```python
from build123d import *

# Parameters (mm, degrees)
BOSS_EXTRUDE2_DEPTH = 2.54
BOSS_EXTRUDE3_DEPTH = 12.7
CUT_EXTRUDE1_DEPTH  = 13.97
FILLET1_R           = 3.8099999999999996


with BuildPart() as part:
    # Sketch1 → Boss-Extrude2 (new body)
    with BuildSketch(Plane(origin=(0, 0, 0), x_dir=(1, 0, 0), z_dir=(0, 1, 0))):
        Polygon((49.12673440534523, 7.27e-15), (24.56336720267261, 42.545), (-24.56336720267263, 42.544999999999995), (-49.12673440534525, -4.56e-15), (-24.56336720267264, -42.545), (24.56336720267261, -42.545), align=None)
        Polygon((-23.09689751893098, 40.004999999999995), (-24.56336720267272, 37.465000000000906), (-21.263810414254024, 35.560000000000905), (-39.522768565701696, 3.9345567884195773), (-38.42291630289545, 3.299556788419578), (-20.163958151447684, 34.925), (-20.163958151447687, 38.735), (16.353958151447667, 38.735), (16.353958151447667, 40.004999999999995), align=None, mode=Mode.SUBTRACT)
        Polygon((20.1639581514492, -34.92499999999734), (38.42291630289649, -3.299556788416705), (39.52276856570363, -3.934556788417227), (21.263810414255218, -35.55999999999977), (24.56336720267305, -37.464999999999264), (23.096897518930962, -40.004999999999995), (-16.353958151447596, -40.0049999999992), (-16.353958151447596, -38.7350000000008), (20.1639581514492, -38.7350000000008), align=None, mode=Mode.SUBTRACT)
        Polygon((40.32791630289463, 1.40742e-12), (22.06895815144691, 31.625443211581366), (23.168810414254217, 32.26044321158198), (41.42776856570169, 0.6350000000010452), (44.727325354119536, 2.540000000000058), (46.19379503786194, 0), (26.468367202673054, -34.16544321158055), (25.368514939866817, -33.53044321158055), (43.62747309131447, -1.9049999999993157), align=None, mode=Mode.SUBTRACT)
        Polygon((20.16395815144767, 34.925), (-16.35395815144768, 34.925), (-16.35395815144768, 36.195), (20.16395815144767, 36.195), (20.163958151447673, 40.004999999999995), (23.096897518930962, 40.004999999999995), (42.82232535411953, 5.839556788418761), (41.7224730913133, 5.204556788418767), (23.4635149398656, 36.83000000000007), align=None, mode=Mode.SUBTRACT)
        Polygon((-40.32791630289535, 3.53e-15), (-22.068958151447685, -31.6254432115805), (-23.168810414253926, -32.26044321158051), (-41.427768565701626, -0.634999999999201), (-44.72732535412034, -2.5399999999991967), (-46.19379503786196, -8.7e-16), (-26.468367202672724, 34.16544321158219), (-25.368514939866504, 33.530443211582195), (-43.62747309131417, 1.9050000000008698), align=None, mode=Mode.SUBTRACT)
        Polygon((-20.163958151444543, -34.92499999999999), (16.35395815144779, -34.924999999999194), (16.353958151447785, -36.19500000000081), (-20.1639581514476, -36.19500000000081), (-20.1639581514476, -40.00499999999919), (-23.09689751893098, -40.004999999999995), (-42.82232535412034, -5.839556788417916), (-41.72247309131411, -5.204556788417918), (-23.46351493986529, -36.83000000000117), align=None, mode=Mode.SUBTRACT)
    extrude(amount=BOSS_EXTRUDE2_DEPTH)

    # Sketch2 → Boss-Extrude3 (add)
    with BuildSketch(Plane(origin=(0, 2.54, 0), x_dir=(1, 0, 0), z_dir=(0, 1, 0))):
        Polygon((-20.163958151447684, 34.925), (-40.32791630289537, -2.429e-14), (-20.163958151447673, -34.92500000000001), (20.163958151447694, -34.92500000000001), (40.32791630289537, 2.74e-15), (20.163958151447677, 34.925), align=None)
    extrude(amount=BOSS_EXTRUDE3_DEPTH)

    # Sketch3 → Cut-Extrude1 (cut)
    with BuildSketch(Plane.XZ):
        Polygon((17.23101878396438, -29.844999999999995), (34.46203756792874, 9.8e-15), (17.231018783964352, 29.845000000000006), (-17.231018783964387, 29.845000000000002), (-34.46203756792876, -6.96e-15), (-17.231018783964384, -29.84499999999999), align=None)
    extrude(amount=-CUT_EXTRUDE1_DEPTH, mode=Mode.SUBTRACT)

    # Fillet1
    fillet1_edges = [part.edges().sort_by_distance(p)[0] for p in [
        (20.163958151447677, 8.89, -34.925),
        (-20.163958151447684, 8.89, -34.925),
        (-40.32791630289537, 8.89, 2.429e-14),
        (-20.163958151447673, 8.89, 34.92500000000001),
        (20.163958151447694, 8.89, 34.92500000000001),
        (40.32791630289537, 8.89, -2.74e-15),
        (-3.55e-15, 15.239999999999998, -34.925),
        (-30.245937227171524, 15.239999999999998, -17.462499999999988),
        (-30.24593722717152, 15.239999999999998, 17.46250000000002),
        (1.066e-14, 15.239999999999998, 34.92500000000001),
        (30.24593722717153, 15.239999999999998, 17.462500000000006),
        (30.245937227171524, 15.239999999999998, -17.462500000000002),
    ]]
    fillet(fillet1_edges, radius=FILLET1_R)


solid = part.part
```
Input: part model. Units: mm. Frame: model coordinates. A direction names the side the tool comes from. Give positions to 0.01 mm unless a question says otherwise; leave off trailing zeros. Order: outer loops, then holes, each group sorted by start corner. A loop starts at its lowest first (then second) coordinate and runs counter-clockwise, first axis right, second up.
1. Section A-A on x = -14.5. Return the cut outline in (y, z) (3 decimals), and give its area (3 significant figures).
Derived:
outline: (0, -42.545) - (2.54, -42.545) - (2.54, -40.005) - (0, -40.005) - close; (0, -38.735) - (2.54, -38.735) - (2.54, -36.195) - (0, -36.195) - close; (0, -34.925) - (11.43, -34.925) arc R3.81 ccw to (15.24, -31.115) - (15.24, 31.115) arc R3.81 ccw to (11.43, 34.925) - (0, 34.925) - (0, 29.845) - (13.97, 29.845) - (13.97, -29.845) - (0, -29.845) - close; (0, 36.195) - (2.54, 36.195) - (2.54, 38.735) - (0, 38.735) - close; (0, 40.005) - (2.54, 40.005) - (2.54, 42.545) - (0, 42.545) - close
area: 250 mm2
2. Reachability of faces 1 (the cylindrical face through (0.251, 14.154, 33.779)), 2 (the flat face through (-2, 1, -38.735)), 3 (the cylindrical face through (19.845, 7.047, -34.428)), 4 (the flat face through (-25.726, 6.887, 15.131)) from +Z, -Z, +X, -X, +Y, -Y: full face, straight path, thin tool, end or side. Return the list, or none.
Derived:
face 1: +Z, +X, -X, +Y
face 2: +Y, -Y
face 3: -Z, +X, +Y
face 4: -Y
3. Pin query (flat end, axial travel): pin 1 (1 mm diameter, centred on y = 1.5, z = -39.5, fed in from -X); pin 2 (1 mm diameter, centred on y = 2, z = -35.5, fed in from +X); pin 3 (1.5 mm diameter, centred on y = 3.5, z = -12.5, fed in from +X). Return the tip coordinate at first contact, or that it passes through.
Derived:
pin 1: stops at x = -26.61
pin 2: stops at x = 28.92
pin 3: stops at x = 33.54
4. Material intervals for L1, parallel to Z at x = -5, y = 4.75 (3 decimals); L2, parallel to Y at x = 14, z = -13; L3, parallel to X at y = 2.5, z = -6.5, sorted ascending.
Derived:
L1: z = -34.925 to -29.845, 29.845 to 34.925
L2: y = 13.97 to 15.24
L3: x = -45.37 to -42.44, -40.97 to -38.04, -36.58 to -30.71, 30.71 to 36.58, 38.04 to 40.97, 42.44 to 45.37
5. Section B-B on y = 6.25. Return the cut outline in (x, z) (1 decimal), and give its area (3 significant figures).
Derived:
outline: (-39.2, -1.9) - (-21.3, -33) arc R3.8 ccw to (-18, -34.9) - (18, -34.9) arc R3.8 ccw to (21.3, -33) - (39.2, -1.9) arc R3.8 ccw to (39.2, 1.9) - (21.3, 33) arc R3.8 ccw to (18, 34.9) - (-18, 34.9) arc R3.8 ccw to (-21.3, 33) - (-39.2, 1.9) arc R3.8 ccw to start; hole (-34.5, 0) - (-17.2, -29.8) - (17.2, -29.8) - (34.5, 0) - (17.2, 29.8) - (-17.2, 29.8) - close
area: 1,140 mm2
6. Section C-C on z = 25. Give the number of separate pieces and of enclosed holes in the cut face, and give its area (3 significant figures).
Derived:
separate pieces: 5
enclosed holes: 0
area: 252 mm2
7. Mould query, pull axis Z, two halves, no side actions, for faces 5 (the flat face through (-1, 15.24, 0)), 6 (the flat face through (0, 1, 42.545)), 7 (the flat face through (2, 1, 38.735)). Classes: released by +Z, released by -Z, zero draft, split by the parting line, or undercut.
Derived:
face 5: zero draft
face 6: released by +Z
face 7: undercut
